Drawing for the job (mm, zero at the part's lowest x, y, z). Coordinates: 2 decimals unless noted, no trailing zeros. Write each loop counter-clockwise with the first axis right and the second up, starting at its lowest first coordinate (ties: lowest second). Pieces come first, ordered by that corner, then holes. Notation, with made-up numbers: (4, 48) -> (52, 48) arc R31 cw to (52, 73) -> close; hole circle Ø4 at (53, 0.25). An arc over 180 degrees is marked (long way). Write item = value, one per line. Start each with the question number.
Q1. Band-saw the part on A-A, the plane z = 20. Give the number of separate pieces and of enclosed holes in the cut face, plus the area to 3 significant figures.
Q2. Pin check, flat tips, straight feed: P1, Ø5, axis at x = 9, y = 8, coming from the +Z side; P2, Ø8, axis at y = 11.5, z = 24, coming from the +X side; P3, Ø5, axis at x = 29, y = 11.5, coming from the +Z side; P4, Ø16, axis at x = 25.88, z = 28.09, coming from the -Y side. Stop position of each tip, or through.
Q3. Pull direction Z, two halves, no side cores. Call the marked faces 1, 2 and 3: released by +Z, released by -Z, zero draft, split by the parting line, or undercut.
Q4. Probe line 1 (Z direction, x = 20, y = 6.25); line 2 (Z direction, x = 20, y = 12.5); line 3 (X direction, y = 6.25, z = 13.5) (1 decimal). List the from-to ranges inside material, lowest first.
Q5. Band-saw the part on B-B, the plane y = 10.75. List the corners of the cut face in (x, z).
Q6. Band-saw the part on D-D, the plane y = 8.25. List the corners of the cut face in (x, z), plus the area to 3 significant figures.
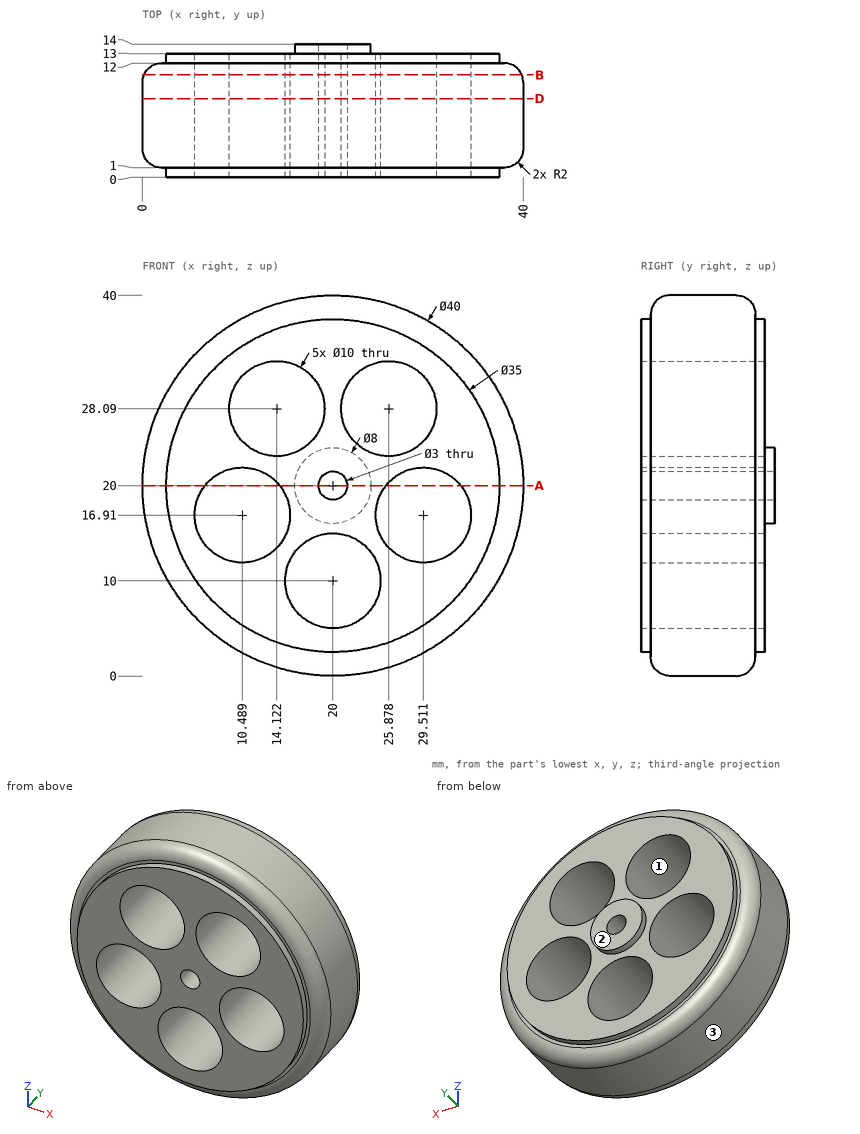
Ans:
q1.separate_pieces = 4
q1.enclosed_holes = 0
q1.area = 268 mm2
q2.P1 = 38.1
q2.P2 = 40
q2.P3 = 38.78
q2.P4 = 0
q3.face_1 = undercut
q3.face_2 = zero draft
q3.face_3 = split by the parting line
q4.line_1 = 0 to 5, 15 to 18.5, 21.5 to 40
q4.line_2 = 2.5 to 5, 15 to 18.5, 21.5 to 37.5
q4.line_3 = 1.1 to 6.8, 14.1 to 16.4, 23.6 to 25.9, 33.2 to 38.9
q5.outline = circle Ø39.71 at (20, 20); hole circle Ø10 at (10.49, 16.91); hole circle Ø10 at (14.12, 28.09); hole circle Ø10 at (20, 10); hole circle Ø3 at (20, 20); hole circle Ø10 at (25.88, 28.09); hole circle Ø10 at (29.51, 16.91)
q6.outline = circle Ø40 at (20, 20); hole circle Ø10 at (10.49, 16.91); hole circle Ø10 at (14.12, 28.09); hole circle Ø10 at (20, 10); hole circle Ø3 at (20, 20); hole circle Ø10 at (25.88, 28.09); hole circle Ø10 at (29.51, 16.91)
q6.area = 857 mm2
